Geometry check sheet. Reference: drawing and pictorial views, mm from the part's lowest x, y, z. A direction names the side the tool comes from. Coordinates: 2 decimals unless noted, no trailing zeros. Loops run counter-clockwise (first coordinate to the right, second up) from the corner with the lowest first, then second, coordinate; pieces in that order, holes last. Notation, with made-up numbers: (20, -26) -> (24, -26) arc R25 ccw to (24, 7) -> close; hole circle Ø7 at (62.25, 60.25). An arc over 180 degrees is marked (long way). Answer as a JSON object with one key per item and string values.
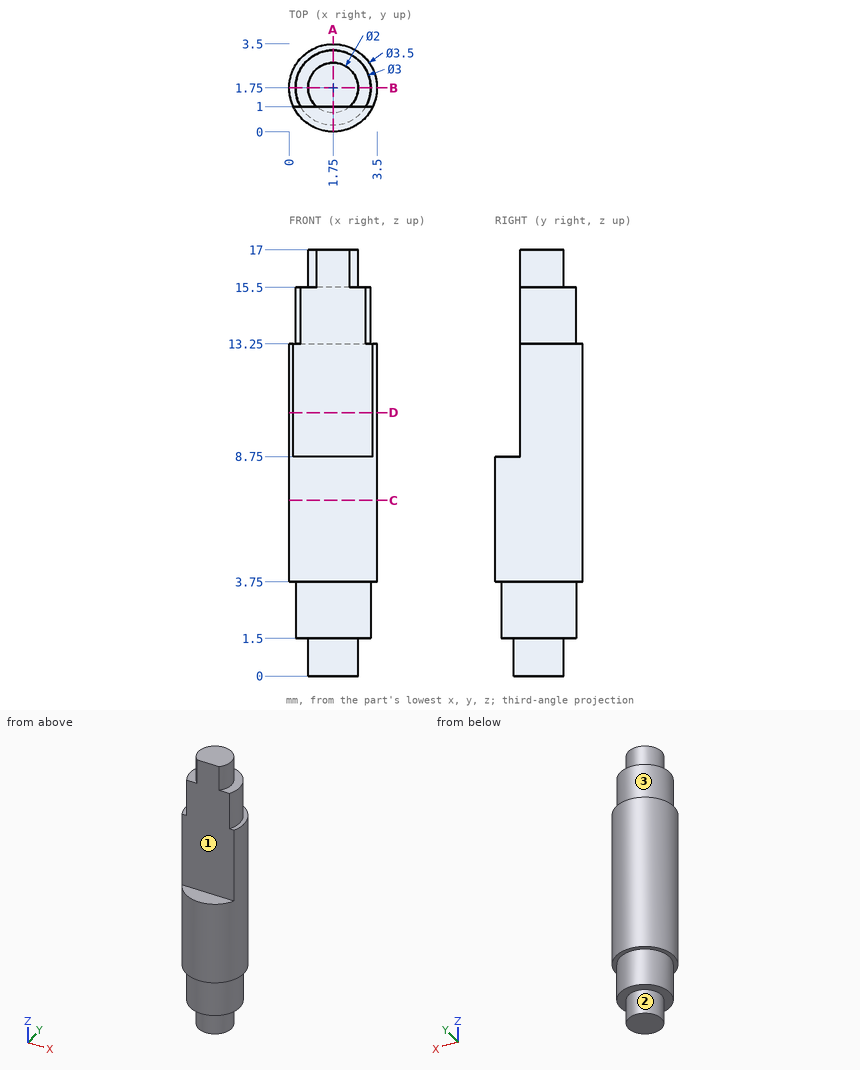
1. Section check B-B, the plane y = 1.75. Record the boundary of the cut face in (x, z), then the cut area to 4 significant figures.
Evaluation:
{"outline": "(0, 3.75) -> (0.25, 3.75) -> (0.25, 1.5) -> (0.75, 1.5) -> (0.75, 0) -> (2.75, 0) -> (2.75, 1.5) -> (3.25, 1.5) -> (3.25, 3.75) -> (3.5, 3.75) -> (3.5, 13.25) -> (3.25, 13.25) -> (3.25, 15.5) -> (2.75, 15.5) -> (2.75, 17) -> (0.75, 17) -> (0.75, 15.5) -> (0.25, 15.5) -> (0.25, 13.25) -> (0, 13.25) -> close", "area": "52.75 mm^2"}
2. Section check C-C, the plane z = 7. Record the boundary of the cut face in (x, y), then the cut area to 3 significant figures.
Evaluation:
{"outline": "circle Ø3.5 at (1.75, 1.75)", "area": "9.62 mm^2"}
3. Tool access check on the marked faces 1, 2 and 3. Record the directions out of +Z, -Z, +X, -X, +Y, -Y that give a thin tool (end or side, any length) a straight path to the whole face; none if there is none.
Evaluation:
{"face 1": "+Z, +X, -X, -Y", "face 2": "-Z", "face 3": "+Z"}
4. Depth check by flat-ended pin: P1, Ø1.6, axis at x = 2, z = 14, coming from the -Y side; P2, Ø1, axis at x = 2.5, z = 8, coming from the -Y side. Enter the tip coordinate at first touch or a pass-through.
Evaluation:
{"P1": "stops at y = 1", "P2": "stops at y = 0.02"}
5. Section check A-A, the plane x = 1.75. Record the boundary of the cut face in (y, z), then the cut area to 3 significant figures.
Evaluation:
{"outline": "(0, 3.75) -> (0.25, 3.75) -> (0.25, 1.5) -> (0.75, 1.5) -> (0.75, 0) -> (2.75, 0) -> (2.75, 1.5) -> (3.25, 1.5) -> (3.25, 3.75) -> (3.5, 3.75) -> (3.5, 13.25) -> (3.25, 13.25) -> (3.25, 15.5) -> (2.75, 15.5) -> (2.75, 17) -> (1, 17) -> (1, 8.75) -> (0, 8.75) -> close", "area": "46.2 mm^2"}
6. Thickness scan on probe 1 along Y at (x, z) = (1, 8); probe 2 along Z at (x, y) = (0.7, 1.7); probe 3 along Y at (x, z) = (1.8, 3.25). Record the ranges inside material, lowest first. Write a range as from..to.
Evaluation:
{"probe 1": "y = 0.17..3.33", "probe 2": "z = 1.5..15.5", "probe 3": "y = 0.25..3.25"}
7. Section check D-D, the plane z = 10.5. Record the boundary of the cut face in (x, y).
Evaluation:
{"outline": "(0.17, 1) -> (3.33, 1) arc R1.75 ccw (long way) to start"}
